```python
from build123d import *

# Parameters (mm, degrees)
ESQUISSE1_R             = 7.5
BOSS_EXTRU_1_DEPTH      = 1.5
ESQUISSE2_W             = 20.2
ESQUISSE2_H             = 20.2
BOSS_EXTRU_2_DEPTH      = 30
ESQUISSE6_R             = 2
ENL_V_MAT_EXTRU_1_DEPTH = 10
CHANFREIN1_SIZE         = 0.3
CONG_1_R                = 2


with BuildPart() as part:
    # Esquisse1 → Boss.-Extru.1 (new body)
    with BuildSketch(Plane.XY):
        Circle(ESQUISSE1_R)
    extrude(amount=BOSS_EXTRU_1_DEPTH)

    # Esquisse2 → Boss.-Extru.2 (add)
    with BuildSketch(Plane(origin=(0, 0, 0), x_dir=(-1, 0, 0), z_dir=(0, 0, -1))):
        Rectangle(ESQUISSE2_W, ESQUISSE2_H)
    extrude(amount=BOSS_EXTRU_2_DEPTH)

    # Esquisse6 → Enlèv. mat.-Extru.1 (cut)
    with BuildSketch(Plane.XY.offset(1.5)):
        Circle(ESQUISSE6_R)
    extrude(amount=-ENL_V_MAT_EXTRU_1_DEPTH, mode=Mode.SUBTRACT)

    # Chanfrein1
    chanfrein1_edges = [part.edges().sort_by_distance(p)[0] for p in [
        (-7.5, 0, 1.5),
    ]]
    chamfer(chanfrein1_edges, length=CHANFREIN1_SIZE)

    # Congé1
    cong_1_edges = [part.edges().sort_by_distance(p)[0] for p in [
        (-10.1, -10.1, -15),
        (-10.1, 10.1, -15),
        (10.1, 10.1, -15),
        (10.1, -10.1, -15),
    ]]
    fillet(cong_1_edges, radius=CONG_1_R)


solid = part.part
```
For this review, take the finished solid that the model builds, in its own axes (mm). A direction names the side the tool comes from. Round coordinates to 2 decimals unless told otherwise and drop trailing zeros. Write each loop counter-clockwise with the first axis right and the second up, starting at its lowest first coordinate (ties: lowest second). Pieces come first, ordered by that corner, then holes. Notation, with made-up numbers: (31, -1) -> (59, -1) arc R19 cw to (59, 26) -> close; hole circle Ø3 at (-35, -5.5). An arc over 180 degrees is marked (long way). One line per question, with ' | ' between items. Start each with the question number.
(1) Mouldability with a two-part tool opening along X and no side actions: class faces 1 (the face through (-7.493, 0.33, 0.592)), 2 (the face through (0, -10.1, -15)), 3 (the face through (0, -2, -3)), 4 (the face through (0, 0, -8.5)) as released by +X, released by -X, zero draft, split by the parting line, or undercut.
(2) For line 1 along Y through (x, z) = (0, -3.5); line 2 along Z through (x, y) = (8, 9.25); line 3 along Z through (x, y) = (0, -1.5), list the stretches that pass through material, from the lowest coordinate up. Write a range as from..to.
(3) Add section C-C, the plane y = 8.5. Write out the cut boundary in (x, z).
(4) Tool access review of faces 5 (the face through (7, 5, 0)), 6 (the face through (10.1, 0, -15)): name each direction out of +Z, -Z, +X, -X, +Y, -Y from which nothing blocks a thin tool from reaching the whole face with its end or side.
(5) Add section A-A, the plane x = 0. Write out the cut boundary in (y, z), plus the area to 3 significant figures.
Answer list:
1) face 1: split by the parting line | face 2: zero draft | face 3: undercut | face 4: undercut
2) line 1: -10.1..-2, 2..10.1 | line 2: -30..0 | line 3: -30..-8.5
3) outline: (-10.06, -30) -> (10.06, -30) -> (10.06, 0) -> (-10.06, 0) -> close
4) face 5: +Z | face 6: +Z, -Z, +X, +Y, -Y
5) outline: (-10.1, -30) -> (10.1, -30) -> (10.1, 0) -> (7.5, 0) -> (7.5, 1.2) -> (7.2, 1.5) -> (2, 1.5) -> (2, -8.5) -> (-2, -8.5) -> (-2, 1.5) -> (-7.2, 1.5) -> (-7.5, 1.2) -> (-7.5, 0) -> (-10.1, 0) -> close | area: 588 mm²
